Part model, mm, in its own coordinate system. A direction names the side the tool comes from. Coordinates: 2 decimals unless noted, no trailing zeros. Loops run counter-clockwise (first coordinate to the right, second up) from the corner with the lowest first, then second, coordinate; pieces in that order, holes last. Notation, with made-up numbers: (43.5, 84.25) - (70.5, 84.25) arc R33 cw to (70.5, 112.25) - close; hole circle Ø7 at (30, 78.25). An arc over 180 degrees is marked (long way). Use a Markdown table: item, result. Add a question column.
1. 3-axis set-ups, long thin cutter, end or side, ignore diameter. For faces 5 (the flat face through (-42.1, 1, 3)), 6 (the flat face through (-4, -43, 6)): which of +Z, -Z, +X, -X, +Y, -Y reach the whole face in a straight line?
2. Wall check: probe 1 along X at (y, z) = (-41, 4.35); probe 2 along Y at (x, z) = (41.5, 0.35); probe 3 along X at (y, z) = (-7, 4.9). Give the ranges that are in metal, low to high. Write a range as [from, to].
3. Band-saw the part on B-B, the plane z = 1.15. Give the cut face in (x, y), plus the area to 3 significant figures.
4. Band-saw the part on A-A, the plane y = 18. Give the cut face in (x, z).
5. Pull direction Y, two halves, no side cores. Call faces 1 (the cylindrical face through (-44.6, 44.67, 2.28)), 2 (the flat face through (-1, -42.1, 3)), 3 (the flat face through (1, 42.1, 3)), 4 (the flat face through (-46.1, 1, 2)): pulls with the +Y half, pulls with the -Y half, needs draft (parallel to the pull), parting line crosses it, or undercut.
Autodesk Fusion 360 part; units mm, degrees
sketch "Sketch1" plane through (0, 0, 0) normal (0, 0, 1) x (1, 0, 0)
  line L0 (42.1, 42.1) -> (-42.1, 42.1)
  line L1 (-42.1, 42.1) -> (-42.1, -42.1)
  line L2 (-42.1, -42.1) -> (42.1, -42.1)
  line L3 (42.1, -42.1) -> (42.1, 42.1)
  line L4 (42.1, 42.1) -> (-42.1, -42.1) construction
  line L5 (-42.1, 42.1) -> (42.1, -42.1) construction
  line L6 (-46.1, -46.1) -> (46.1, -46.1)
  line L7 (46.1, -46.1) -> (46.1, 46.1)
  line L8 (46.1, 46.1) -> (-46.1, 46.1)
  line L9 (-46.1, 46.1) -> (-46.1, -46.1)
  dimension "d1" = 84.2
  dimension "d2" = 84.2
  dimension "d3" = 4
extrude "Extrude1" add sketch "Sketch1" along normal blind 6
fillet "Fillet1" radius 5 4 edges at (-46.1, -46.1, 3) (46.1, -46.1, 3) (46.1, 46.1, 3) (-46.1, 46.1, 3)
fillet "Fillet2" radius 1.5 8 edges at (-44.6355, 44.6355, 6) (-46.1, 0, 6) (-44.6355, -44.6355, 6) (0, -46.1, 6) (44.6355, -44.6355, 6) (46.1, 0, 6) (44.6355, 44.6355, 6) (0, 46.1, 6)
Geometry check:
| question | item | result |
|---|---|---|
| 1 | face 5 | +Z, -Z |
| 1 | face 6 | +Z, +X, -X, +Y, -Y |
| 2 | probe 1 | x = [-46.1, -42.1], [42.1, 46.1] |
| 2 | probe 2 | y = [-46.08, -42.1], [42.1, 46.08] |
| 2 | probe 3 | x = [-46.05, -42.1], [42.1, 46.05] |
| 3 | outline | (-46.1, -41.1) arc R5 ccw to (-41.1, -46.1) - (41.1, -46.1) arc R5 ccw to (46.1, -41.1) - (46.1, 41.1) arc R5 ccw to (41.1, 46.1) - (-41.1, 46.1) arc R5 ccw to (-46.1, 41.1) - close; hole (-42.1, -42.1) - (42.1, -42.1) - (42.1, 42.1) - (-42.1, 42.1) - close |
| 3 | area | 1,390 mm^2 |
| 4 | outline | (-46.1, 0) - (-42.1, 0) - (-42.1, 6) - (-44.6, 6) arc R1.5 ccw to (-46.1, 4.5) - close; (42.1, 0) - (46.1, 0) - (46.1, 4.5) arc R1.5 ccw to (44.6, 6) - (42.1, 6) - close |
| 5 | face 1 | pulls with the +Y half |
| 5 | face 2 | undercut |
| 5 | face 3 | undercut |
| 5 | face 4 | needs draft |
